Can you work these out from the model? Positions are in its coordinate system, mm. A direction names the side the tool comes from. Coordinates: 2 decimals unless noted, no trailing zeros. Write each loop counter-clockwise with the first axis right and the second up, starting at its lowest first coordinate (ties: lowest second). Pieces come first, ordered by that corner, then holes. Notation, with made-up numbers: (59, 45) -> (88, 45) arc R18 cw to (88, 71) -> close; hole circle Ø3 at (88.25, -7). An arc over 180 degrees is marked (long way). Use one line per item in the form item = value.
Autodesk Inventor part; units mm, degrees
ref_plane "РабПлоскость1" through (0, 0, -80) normal (0, 0, 1) x (1, 0, 0)
ref_plane "YZ Plane" through (0, 0, 0) normal (1, 0, 0) x (0, 1, 0)
ref_plane "XZ Plane" through (0, 0, 0) normal (0, 1, 0) x (-1, 0, 0)
sketch "Эскиз1" plane through (0, 0, 0) normal (0, 0, 1) x (1, 0, 0)
  line L0 (-42.5, 0) -> (-13.1332, 40.4199)
  line L1 (-13.1332, 40.4199) -> (34.3832, 24.9809)
  line L2 (34.3832, 24.9809) -> (34.3832, -24.9809)
  line L3 (34.3832, -24.9809) -> (-13.1332, -40.4199)
  line L4 (-13.1332, -40.4199) -> (-42.5, 0)
  point P0 (0, 0)
  point P1 (0, 0)
sketch "Эскиз2" plane through (0, 0, 0) normal (0, 1, 0) x (-1, 0, 0)
  line L0 (30, -10) -> (-20, -10)
  line L1 (-20, -10) -> (-10, -40)
  line L2 (-10, -40) -> (15, -40)
  line L3 (15, -40) -> (30, -10)
  line L4 (13.1332, 0) -> (-34.3832, 0)
  line L5 (42.5, 0) -> (13.1332, 0)
  point P0 (0, 0)
  dimension "d1" = 10
  dimension "d2" = 30
  dimension "d3" = 10
  dimension "d4" = 20
  dimension "d5" = 50
  dimension "d6" = 25
ref_plane "РабПлоскость1" through (0, 0, -80) normal (0, 0, 1) x (1, 0, 0)
sketch "Эскиз3" plane through (0, 0, -80) normal (0, 0, 1) x (1, 0, 0)
  point P0 (0, 0)
  point P1 (0, 0)
  point P2 (0, 0)
loft "Лофт1" add profiles "Эскиз1" section 2 point at (0, 0, -80)
extrude "Выдавливание1" cut sketch "Эскиз2" along normal through all both and the other way through all
properties part number "Шар"
Q1. For faces 4 (the flat face through (15.55, -18.295, -28.335)), 5 (the flat face through (-2, 0, -40)), which set-ups out of +Z, -Z, +X, -X, +Y, -Y let a thin tool reach every point of the face, with its end or its side?
Return value:
face_4 = -Z, +X, -Y
face_5 = +Y, -Y
Q2. Suppose I cut it at B-B (y = 17). Write out the boundary of the cut face in (x, z).
Return value:
outline = (-30.15, 0) -> (-24.84, -10) -> (20, -10) -> (12.11, -33.68) -> (23.4, -25.56) -> (34.38, 0) -> close; (-8.9, -40) -> (-5.52, -46.35) -> (3.31, -40) -> close
Q3. Suppose I cut it at C-C (x = 5.5). Write out the boundary of the cut face in (y, z), then the cut area to 3 significant figures.
Return value:
outline = (-34.37, 0) -> (-29.85, -10) -> (29.85, -10) -> (34.37, 0) -> close; (-16.29, -40) -> (-4, -67.2) -> (4, -67.2) -> (16.29, -40) -> close
area = 1,190 mm2
Q4. Suppose I cut it at A-A (z = -21.5). Write out the boundary of the cut face in (x, y), then the cut area to 3 significant figures.
Return value:
outline = (-31.08, 0) -> (-24.25, -9.4) -> (-24.25, 9.4) -> close; (16.17, -21.18) -> (25.14, -18.27) -> (25.14, 18.27) -> (16.17, 21.18) -> close
area = 418 mm2
Q5. Thinking about a two-plate mould opening in X: for faces 1 (the flat face through (-2, 3, 0)), 2 (the flat face through (20.77, -0.35, -31.67)), 3 (the flat face through (-22.4, -0.1, -25.2)), which applies, released by +X, released by -X, zero draft, split by the parting line, or undercut?
Return value:
face_1 = zero draft
face_2 = released by +X
face_3 = undercut
Q6. Will these pins go through, and if not, where does the flat tip stop? pin 1 (2 mm diameter, centred on x = 2.5, y = 27.5, fed in from +Z); pin 2 (10 mm diameter, centred on y = -8.5, z = -42, fed in from +X); pin 3 (10 mm diameter, centred on x = 7, y = -23.5, fed in from -Z); pin 4 (1.5 mm diameter, centred on x = -2, z = -49, fed in from -Y).
Return value:
pin_1 = 0
pin_2 = 18.48
pin_3 = -10
pin_4 = -15.08
Q7. Suppose I cut it at D-D (y = -6.5). Write out the boundary of the cut face in (x, z).
Return value:
outline = (-37.78, 0) -> (-2.11, -67.14) -> (8.95, -59.18) -> (34.38, 0) -> close; hole (-30, -10) -> (-15, -40) -> (10, -40) -> (20, -10) -> close
Q8. If I drill on line 1 (X direction, y = -2.5, z = -19.5); line 2 (Z direction, x = 2, y = 22.5); line 3 (Z direction, x = -3.5, y = 15.5), over which ranges is the centre line in solid material (lowest first)? Write a range as from..to.
Return value:
line_1 = -30.32..-25.25, 16.83..26
line_2 = -10..0
line_3 = -48.22..-40, -10..0
